Can you work these out from the model? Positions are in its coordinate system, mm. Face numbers are marked on the shaded views. A direction names the side the tool comes from. Give positions to 0.01 mm unless a question says otherwise; leave off trailing zeros. Loops run counter-clockwise (first coordinate to the right, second up) from the corner with the lowest first, then second, coordinate; pieces in that order, holes last. Notation, with made-up numbers: M 58,73 L 66,73 A18 ccw 66,90 Z; hole C 63,67 d7. An arc over 180 degrees is marked long. Use CSV: the item, a comma, the result in double quotes.
from build123d import *

# Parameters (mm, degrees)
F0_R     = 23.1
F1_DEPTH = 12.5
F2_R     = 20.6
F3_DEPTH = 50
F4_R     = 19.35
F5_DEPTH = 10
F6_T     = -2.5


with BuildPart() as f1:
    # F0 (on Top) → F1 (new body)
    with BuildSketch(Plane.XY):
        Circle(F0_R)
    extrude(amount=F1_DEPTH)

    # F2 (on face) → F3 (join)
    with BuildSketch(Plane.XY.offset(12.5)):
        Circle(F2_R)
    extrude(amount=F3_DEPTH)

    # F4 (on face) → F5 (join)
    with BuildSketch(Plane.XY.offset(62.5)):
        Circle(F4_R)
    extrude(amount=F5_DEPTH)

    # F6
    f6_openings = [f1.faces().sort_by_distance(p)[0] for p in [
        (0, 0, 72.5),
        (0, 0, 0),
    ]]
    offset(amount=F6_T, openings=f6_openings, kind=Kind.INTERSECTION)


solid = f1.part
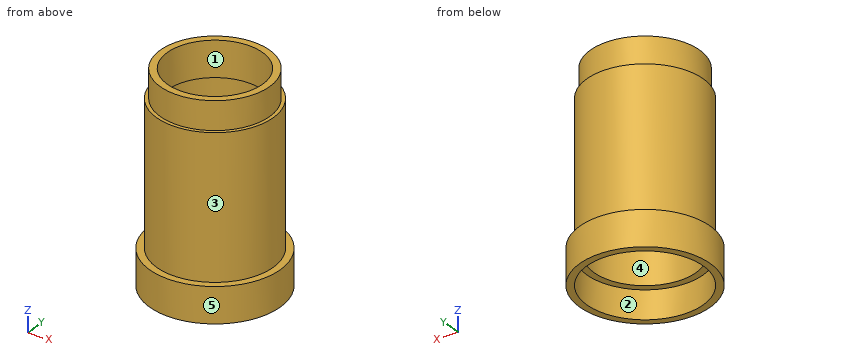
Q1. Please list where these lines run through material, in increasing order: L1, parallel to Y at x = 0, z = 47.5; L2, parallel to Y at x = 0, z = 62; L3, parallel to Z at x = 13.5, y = -15. Write a range as from..to.
Model answer:
L1,"-20.6..-18.1, 18.1..20.6"
L2,"-20.6..-16.85, 16.85..20.6"
L3,"10..62.5"
Q2. I want a section at A-A, the plane y = 0. Please give me the cut outline in (x, z), then the cut area to 3 significant figures.
Model answer:
outline,"M -23.1,0 L -20.6,0 L -20.6,10 L -18.1,10 L -18.1,60 L -16.85,60 L -16.85,72.5 L -19.35,72.5 L -19.35,62.5 L -20.6,62.5 L -20.6,12.5 L -23.1,12.5 Z; M 16.85,60 L 18.1,60 L 18.1,10 L 20.6,10 L 20.6,0 L 23.1,0 L 23.1,12.5 L 20.6,12.5 L 20.6,62.5 L 19.35,62.5 L 19.35,72.5 L 16.85,72.5 Z"
area,"381 mm2"
Q3. For the marked faces 1, 2 and 3, which set-ups out of +Z, -Z, +X, -X, +Y, -Y let a thin tool reach every point of the face, with its end or its side?
Model answer:
face 1,"+Z, -Z"
face 2,"-Z"
face 3,"+Z"
Q4. I want a section at C-C, the plane z = 6. Please give me the cut outline in (x, y), then the cut area to 3 significant figures.
Model answer:
outline,"C 0,0 d46.2; hole C 0,0 d41.2"
area,"343 mm2"
Q5. If we mould it in two halves opening along X, with no side actions, what happens to the marked faces 4 and 5? For each: released by +X, released by -X, zero draft, split by the parting line, or undercut.
Model answer:
face 4,"undercut"
face 5,"split by the parting line"
Q6. I'm going to push flat-ended pins straight in: P1, Ø3, axis at x = -4, y = 17, coming from the -Z side; P2, Ø1.5, axis at y = 4.5, z = 10.5, coming from the -X side; P3, Ø20.5, axis at x = 0, y = -2, coming from the -Z side; P4, Ø8, axis at y = -18, z = 15.5, coming from the +X side. Where does each tip first touch, or does it pass through?
Model answer:
P1,"z = 10"
P2,"x = -22.79"
P3,"through"
P4,"x = 17.26"
Q7. I want a section at D-D, the plane z = 44. Please give me the cut outline in (x, y).
Model answer:
outline,"C 0,0 d41.2; hole C 0,0 d36.2"
